Input: part model. Units: mm. Frame: model coordinates. Face numbers are marked on the shaded views. Round coordinates to 2 decimals unless told otherwise and drop trailing zeros. Loops run counter-clockwise (first coordinate to the right, second up) from the corner with the lowest first, then second, coordinate; pieces in that order, holes last. Notation, with made-up numbers: (40.25, 54) -> (57.25, 54) arc R16 cw to (57.25, 67) -> close; hole circle Ø7 at (-11, 79). An arc over 180 degrees is marked (long way). Answer as a JSON object with one key per item and string values. Group by question number.
Item 1: Section query C-C on z = 8. Return loops of the section in (x, y).
Item 2: Draft query along Z for the marked faces 1, 2 and 3. Return one class per face: released by +Z, released by -Z, zero draft, split by the parting line, or undercut.
Item 3: Section query B-B on y = -15.25. Return loops of the section in (x, z), and give its area (3 significant figures).
Item 4: Section query A-A on x = 33. Return loops of the section in (y, z).
Item 5: Section query D-D on y = -9. Return loops of the section in (x, z), and give its area (3 significant figures).
Item 6: Material intervals for line 1 (X direction, y = -9, z = 1.2); line 2 (Z direction, x = 32.5, y = -15.5); line 3 (Y direction, x = 33, z = 1.7), sorted ascending. Write a range as [from, to].
Item 7: Pin query (flat end, axial travel): pin 1 (5 mm diameter, centred on x = 33, y = -9, fed in from -Z). Return the tip coordinate at first contact, or that it passes through.
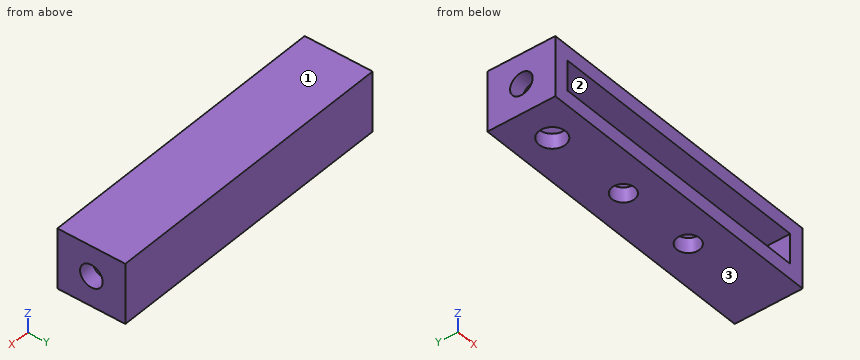
from build123d import *

# Parameters (mm, degrees)
F0_W     = 80
F0_H     = 16
F0_W_2   = 72
F0_H_2   = 8
F1_DEPTH = 18
F2_R     = 3
F3_DEPTH = 80
F4_DEPTH = 4
F5_R     = 3.5
F5_R_2   = 3
F6_DEPTH = 5


with BuildPart() as f1:
    # F0 (on Front) → F1 (new body)
    with BuildSketch(Plane.XZ):
        with Locations((40, 8)):
            Rectangle(F0_W, F0_H)
        with Locations((40, 8)):
            Rectangle(F0_W_2, F0_H_2, mode=Mode.SUBTRACT)
    extrude(amount=F1_DEPTH)

    # F2 (on face) → F3 (cut)
    with BuildSketch(Plane(origin=(0, 0, 0), x_dir=(0, -1, 0), z_dir=(-1, 0, 0))):
        with Locations((9, 8)):
            Circle(F2_R)
    extrude(amount=-F3_DEPTH, mode=Mode.SUBTRACT)

    # F0 (on Front) → F4 (join)
    with BuildSketch(Plane.XZ):
        with Locations((40, 8)):
            Rectangle(F0_W_2, F0_H_2)
    extrude(amount=F4_DEPTH)

    # F5 (on face) → F6 (cut)
    with BuildSketch(Plane(origin=(0, 0, 0), x_dir=(1, 0, 0), z_dir=(0, 0, -1))):
        with Locations((10, 9)):
            Circle(F5_R)
        with Locations((33, 9)):
            Circle(F5_R_2)
        with Locations((54, 9)):
            Circle(F5_R_2)
    extrude(amount=-F6_DEPTH, mode=Mode.SUBTRACT)


solid = f1.part
Solved:
{
 "1": {"outline": "(0, -18) -> (4, -18) -> (4, -12) -> (0, -12) -> close; (0, -6) -> (4, -6) -> (4, -4) -> (76, -4) -> (76, -6) -> (80, -6) -> (80, 0) -> (0, 0) -> close; (76, -18) -> (80, -18) -> (80, -12) -> (76, -12) -> close"},
 "2": {"face 1": "released by +Z", "face 2": "undercut", "face 3": "released by -Z"},
 "3": {"outline": "(0, 0) -> (80, 0) -> (80, 16) -> (0, 16) -> close; hole (4, 4) -> (76, 4) -> (76, 12) -> (4, 12) -> close", "area": "704 mm²"},
 "4": {"outline": "(-18, 0) -> (-12, 0) -> (-12, 4) -> (-18, 4) -> close; (-18, 12) -> (-4, 12) -> (-4, 4) -> (-6, 4) -> (-6, 0) -> (0, 0) -> (0, 16) -> (-18, 16) -> close"},
 "5": {"outline": "(0, 0) -> (6.5, 0) -> (6.5, 4) -> (4, 4) -> (4, 5) -> (0, 5) -> close; (0, 11) -> (4, 11) -> (4, 12) -> (76, 12) -> (76, 11) -> (80, 11) -> (80, 16) -> (0, 16) -> close; (13.5, 0) -> (30, 0) -> (30, 4) -> (13.5, 4) -> close; (36, 0) -> (51, 0) -> (51, 4) -> (36, 4) -> close; (57, 0) -> (80, 0) -> (80, 5) -> (76, 5) -> (76, 4) -> (57, 4) -> close", "area": "580 mm²"},
 "6": {"line 1": "[0, 6.5], [13.5, 30], [36, 51], [57, 80]", "line 2": "[0, 4], [12, 16]", "line 3": "[-18, -12], [-6, 0]"},
 "7": {"pin 1": "z = 12"}
}
